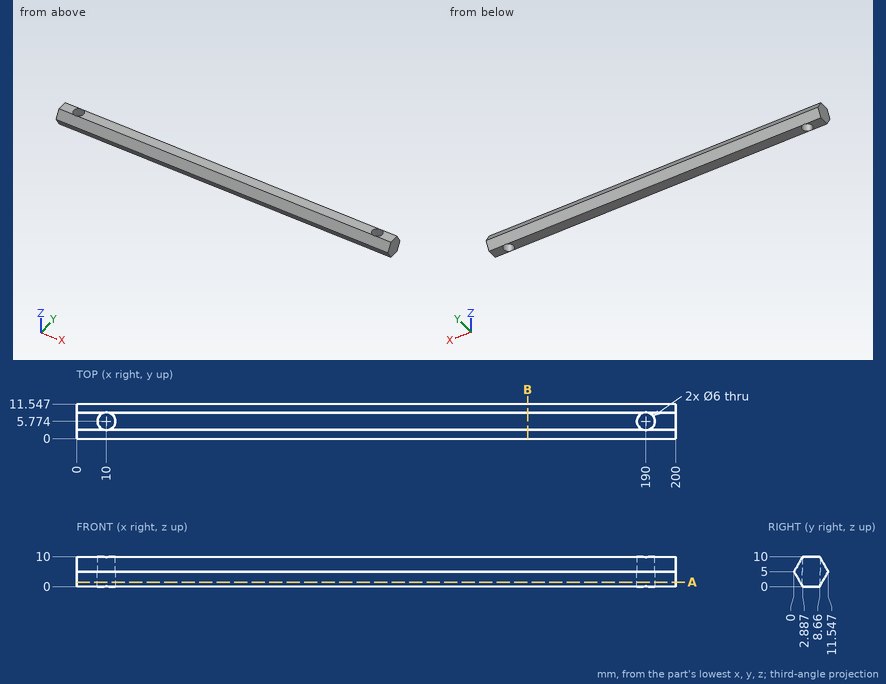
Study the drawing (mm; zero at the part's minimum x, y, z) and answer. Give positions to 0.01 mm unless a question says otherwise; leave off trailing zeros. Loops run counter-clockwise (first coordinate to the right, second up) from the corner with the lowest first, then second, coordinate; pieces in that order, holes last. Notation, with made-up numbers: M 84,70 L 139,70 A16 cw 139,96 Z; hole C 62.5,17 d7. An arc over 180 degrees is marked long. One line per item, written item: value.
1. Each of these flat-tipped pins is pushed along its axis until it touches: P1, Ø1, axis at x = 146.5, z = 2, coming from the -Y side; P2, Ø5, axis at x = 10, y = 5.77, coming from the +Z side; P3, Ø4, axis at x = 68, z = 2, coming from the -Y side. Where does it stop, or does it pass through?
Found:
P1: y = 1.44
P2: through
P3: y = 0.58
2. Section B-B on x = 150.5 is taken. Determine the outline of the cut face in (y, z), plus the area to 3 significant figures.
Found:
outline: M 0,5 L 2.89,0 L 8.66,0 L 11.55,5 L 8.66,10 L 2.89,10 Z
area: 86.6 mm^2
3. Section A-A on z = 1.5 is taken. Determine the outline of the cut face in (x, y).
Found:
outline: M 0,2.02 L 200,2.02 L 200,9.53 L 0,9.53 Z; hole C 10,5.77 d6; hole C 190,5.77 d6
4. Find the intervals of material crossed by probe 1 along X at (y, z) = (5.5, 4.25); probe 2 along X at (y, z) = (6.75, 1.25) (1 decimal); probe 3 along Y at (x, z) = (10, 8.3) (1 decimal), in increasing order.
Found:
probe 1: 0 to 7.01, 12.99 to 187.01, 192.99 to 200
probe 2: 0 to 7.2, 12.8 to 187.2, 192.8 to 200
probe 3: 1.9 to 2.8, 8.8 to 9.6
